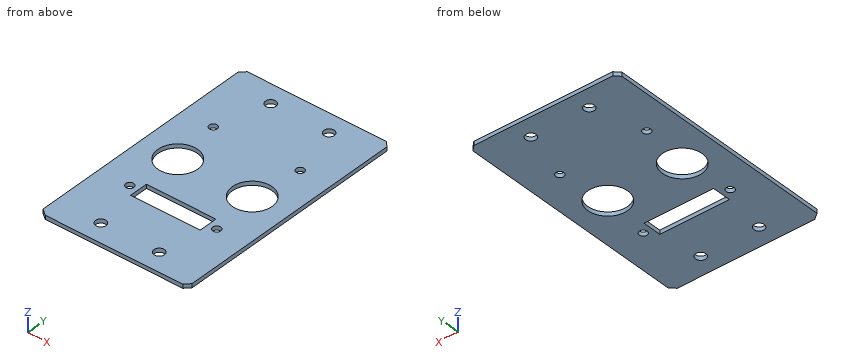
```python
from build123d import *

# Parameters (mm, degrees)
SKETCH_1_R      = 8
SKETCH_1_R_2    = 1.6
SKETCH_1_R_3    = 2.1
SKETCH_1_W      = 28
SKETCH_1_H      = 7.5
EXTRUDE_1_DEPTH = 1.6


with BuildPart() as part:
    # 草图1 → 凸台-拉伸1 (new body)
    with BuildSketch(Plane.XY):
        Polygon((-28, 48.5), (28, 48.5), (30, 46.5), (30, -46.5), (28, -48.5), (-27.38960578, -48.5), (-30, -46.5), (-30, 46.5), align=None)
        with Locations((-15, 0)):
            Circle(SKETCH_1_R, mode=Mode.SUBTRACT)
        with Locations((-17.5, 19.9)):
            Circle(SKETCH_1_R_2, mode=Mode.SUBTRACT)
        with Locations((-11.75, 40.5)):
            Circle(SKETCH_1_R_3, mode=Mode.SUBTRACT)
        with Locations(Location((-17.5, -19.9, 0), (0, 0, 180))):
            Circle(SKETCH_1_R_2, mode=Mode.SUBTRACT)
        with Locations(Location((-11.75, -40.5, 0), (0, 0, 180))):
            Circle(SKETCH_1_R_3, mode=Mode.SUBTRACT)
        with Locations(Location((17.5, 19.9, 0), (0, 0, 180))):
            Circle(SKETCH_1_R_2, mode=Mode.SUBTRACT)
        with Locations(Location((11.75, 40.5, 0), (0, 0, 180))):
            Circle(SKETCH_1_R_3, mode=Mode.SUBTRACT)
        with Locations((11.75, -40.5)):
            Circle(SKETCH_1_R_3, mode=Mode.SUBTRACT)
        with Locations((17.5, -19.9)):
            Circle(SKETCH_1_R_2, mode=Mode.SUBTRACT)
        with Locations(Location((15, 0, 0), (0, 0, 180))):
            Circle(SKETCH_1_R, mode=Mode.SUBTRACT)
        with Locations((0, -19.9)):
            Rectangle(SKETCH_1_W, SKETCH_1_H, mode=Mode.SUBTRACT)
    extrude(amount=EXTRUDE_1_DEPTH)


solid = part.part
```
Input: part model. Units: mm. Frame: model coordinates. Give positions to 0.01 mm unless a question says otherwise; leave off trailing zeros. Loops run counter-clockwise (first coordinate to the right, second up) from the corner with the lowest first, then second, coordinate; pieces in that order, holes last. Notation, with made-up numbers: M -4,23 L 15,23 A23 ccw 15,43 Z; hole C -14,85.25 d11. An arc over 180 degrees is marked long. Answer as CSV lines item,"result". Start each with the question number.
1. Pin query (flat end, axial travel): P1, Ø4, axis at x = 17.5, y = -19.9, coming from the +Z side; P2, Ø1.9, axis at x = -17.5, y = -19.9, coming from the +Z side. Return the tip coordinate at first contact, or that it passes through.
2. Line query: L1, parallel to Y at x = -15, z = 1.25; L2, parallel to Y at x = -11.75, z = 0.45; L3, parallel to X at y = -4, z = 0.65. Output: solid intervals per line, ascending.
3. Section C-C on y = 0. Return loops of the section in (x, z), plus the area to 3 significant figures.
4. Section D-D on z = 1.1. State how many separate pieces and enclosed holes the cut face has, plus the area to 3 significant figures.
5. Section A-A on y = -19.9. Return loops of the section in (x, z), plus the area to 3 significant figures.
6. Section B-B on x = -2.5. Return loops of the section in (y, z).
Computed values:
1,P1,"stops at z = 1.6"
1,P2,"passes through"
2,L1,"y = -48.5 to -8, 8 to 48.5"
2,L2,"y = -48.5 to -42.6, -38.4 to -23.65, -16.15 to -7.31, 7.31 to 38.4, 42.6 to 48.5"
2,L3,"x = -30 to -21.93, -8.07 to 8.07, 21.93 to 30"
3,outline,"M -30,0 L -23,0 L -23,1.6 L -30,1.6 Z; M -7,0 L 7,0 L 7,1.6 L -7,1.6 Z; M 23,0 L 30,0 L 30,1.6 L 23,1.6 Z"
3,area,"44.8 mm²"
4,separate pieces,"1"
4,enclosed holes,"11"
4,area,"5,110 mm²"
5,outline,"M -30,0 L -19.1,0 L -19.1,1.6 L -30,1.6 Z; M -15.9,0 L -14,0 L -14,1.6 L -15.9,1.6 Z; M 14,0 L 15.9,0 L 15.9,1.6 L 14,1.6 Z; M 19.1,0 L 30,0 L 30,1.6 L 19.1,1.6 Z"
5,area,"41.0 mm²"
6,outline,"M -48.5,0 L -23.65,0 L -23.65,1.6 L -48.5,1.6 Z; M -16.15,0 L 48.5,0 L 48.5,1.6 L -16.15,1.6 Z"
